The listing builds one solid part. Answer for the finished solid, in the listing's coordinates (mm). Face numbers are marked on the shaded views. Give positions to 0.01 mm unless a question says otherwise; leave off trailing zeros. Loops run counter-clockwise (first coordinate to the right, second up) from the corner with the lowest first, then second, coordinate; pieces in that order, holes last. Notation, with made-up numbers: M 84,23.25 L 128,23.25 A21 cw 128,57.25 Z; hole C 75.5,17 d7. An arc over 180 degrees is marked long. Return JSON: item names as keys, results as strings.
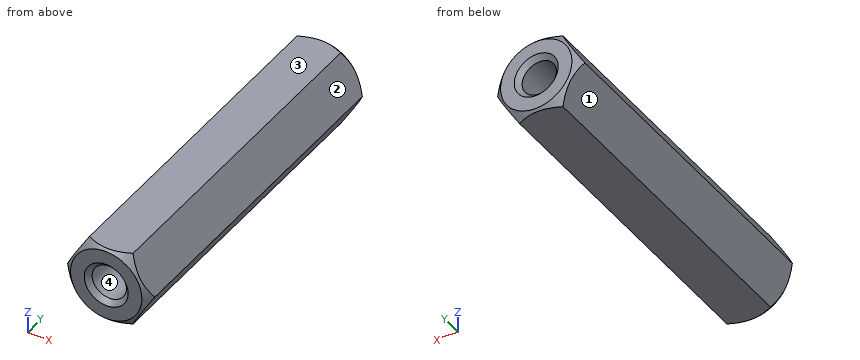
from build123d import *

# Parameters (mm, degrees)
BOSS_EXTRUDE1_DEPTH = 25


with BuildPart() as part:
    # Sketch1 → Boss-Extrude1 (new body)
    with BuildSketch(Plane(origin=(0, 0, 0), x_dir=(1, 0, 0), z_dir=(0, 1, 0))):
        Polygon((1.58771324, 2.75), (-1.58771324, 2.75), (-3.175426481, 0), (-1.58771324, -2.75), (1.58771324, -2.75), (3.175426481, 0), align=None)
    extrude(amount=BOSS_EXTRUDE1_DEPTH)

    # Sketch2 → M3 Tapped Hole1 (revolve, cut)
    with BuildSketch(Plane(origin=(0, 25, 0), x_dir=(0, 0, 1), z_dir=(1, 0, 0))):
        Polygon((0, 0), (0, 25), (1.6, 25), (1.25, 24.65), (1.25, 0.35), (1.6, 0), align=None)
    revolve(axis=Axis((0, 31.35, 0), (0, -1, 0)), mode=Mode.SUBTRACT)

    # Sketch4 → Cut-Revolve1 (revolve, cut)
    with BuildSketch(Plane.XY):
        Polygon((2.6, 0), (3.175426481, 0.575426481), (3.175426481, 0), align=None)
        Polygon((3.175426481, 25), (2.6, 25), (3.175426481, 24.424573519), align=None)
    revolve(axis=Axis((0, 25, 0), (0, -1, 0)), mode=Mode.SUBTRACT)


solid = part.part
(1) The part is cut by section B-B (y = 3.5). Determine the outline of the cut face in (x, z), and give its area (3 significant figures).
Values follow:
{"outline": "M -3.18,0 L -1.59,-2.75 L 1.59,-2.75 L 3.18,0 L 1.59,2.75 L -1.59,2.75 Z; hole C 0,0 d2.5", "area": "21.3 mm²"}
(2) Straight lines are drawn through the part: line 1 along Z through (x, y) = (0, 7.5); line 2 along X through (y, z) = (6.25, 0.8); line 3 along X through (y, z) = (18.25, 0.55). For each, find the intervals that lie inside material, in ascending order.
Values follow:
{"line 1": "-2.75 to -1.25, 1.25 to 2.75", "line 2": "-2.71 to -0.96, 0.96 to 2.71", "line 3": "-2.86 to -1.12, 1.12 to 2.86"}
(3) Determine the mould class of the marked faces 1, 2, 3 and 4 for opening direction X: released by +X, released by -X, zero draft, split by the parting line, or undercut.
Values follow:
{"face 1": "released by -X", "face 2": "released by +X", "face 3": "zero draft", "face 4": "undercut"}
(4) The part is cut by section A-A (x = 0). Determine the outline of the cut face in (y, z).
Values follow:
{"outline": "M 0,-2.6 L 0.15,-2.75 L 24.85,-2.75 L 25,-2.6 L 25,-1.6 L 24.65,-1.25 L 0.35,-1.25 L 0,-1.6 Z; M 0,1.6 L 0.35,1.25 L 24.65,1.25 L 25,1.6 L 25,2.6 L 24.85,2.75 L 0.15,2.75 L 0,2.6 Z"}
(5) Given pin 1 (1.5 mm diameter, centred on y = 18, z = -1, fed in from -X); pin 2 (1 mm diameter, centred on x = -1, z = 0, fed in from -Y); pin 3 (1 mm diameter, centred on x = -0.5, z = 0.5, fed in from -Y), each flat-ended and moving along its own axis, determine where each tip first touches the part or whether it passes through.
Values follow:
{"pin 1": "x = -3.03", "pin 2": "y = 0.1", "pin 3": "through"}
